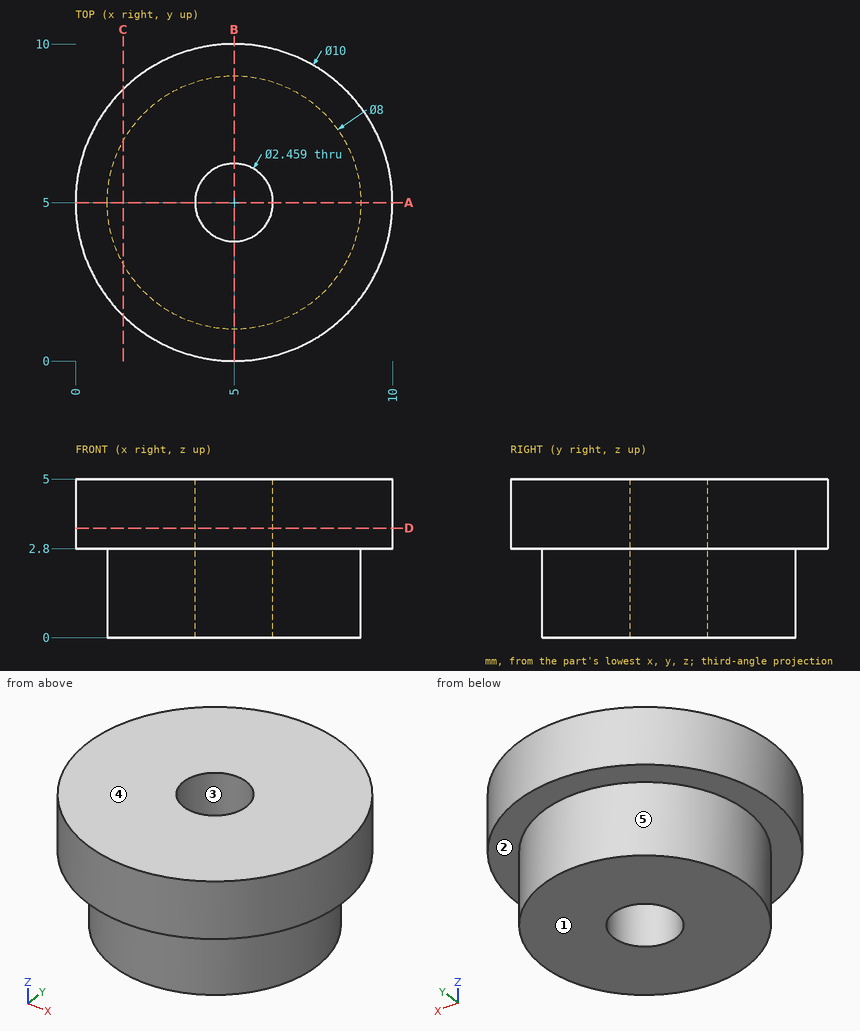
Job drawing, mm, ordinate dimensions from the low corner. One solid piece. A direction names the side the tool comes from. Coordinates: 2 decimals unless noted, no trailing zeros. Loops run counter-clockwise (first coordinate to the right, second up) from the corner with the lowest first, then second, coordinate; pieces in that order, holes last. Notation, with made-up numbers: (73, -26) -> (81, -26) arc R17 ccw to (81, -20) -> close; hole circle Ø1 at (45, 53). An arc over 180 degrees is marked (long way). One line per item, written item: value.
1. Slice it at C-C on x = 1.5. Write the cut outline in (y, z).
Answers:
outline: (1.43, 2.8) -> (3.06, 2.8) -> (3.06, 0) -> (6.94, 0) -> (6.94, 2.8) -> (8.57, 2.8) -> (8.57, 5) -> (1.43, 5) -> close
2. Slice it at A-A on y = 5. Write the cut outline in (x, z), and give its area (3 significant figures).
Answers:
outline: (0, 2.8) -> (1, 2.8) -> (1, 0) -> (3.77, 0) -> (3.77, 5) -> (0, 5) -> close; (6.23, 0) -> (9, 0) -> (9, 2.8) -> (10, 2.8) -> (10, 5) -> (6.23, 5) -> close
area: 32.1 mm^2
3. Pull direction Y, two halves, no side cores. Call the marked faces 3, 4 and 5: pulls with the +Y half, pulls with the -Y half, needs draft (parallel to the pull), parting line crosses it, or undercut.
Answers:
face 3: undercut
face 4: needs draft
face 5: parting line crosses it
4. Which spindle directions (+Z, -Z, +X, -X, +Y, -Y) get a long thin tool onto all of the face, cutting with end or side? Do the marked faces 1 and 2. Say none if no direction does.
Answers:
face 1: -Z, +X, -X, +Y, -Y
face 2: -Z
5. Slice it at D-D on z = 3.45. Write the cut outline in (x, y), and give its area (3 significant figures).
Answers:
outline: circle Ø10 at (5, 5); hole circle Ø2.46 at (5, 5)
area: 73.8 mm^2
6. Flat gauge pins, fed straight in: P1, Ø1.5, axis at y = 7, z = 2.5, coming from the +X side; P2, Ø2, axis at x = 1.5, z = 0.5, coming from the -Y side; P3, Ø1.5, axis at x = 5, y = 5, coming from the +Z side. Where does each tip first touch, or does it go through?
Answers:
P1: stops at x = 9.82
P2: stops at y = 1.88
P3: passes through
7. Drill centre lines: line 1 (Y direction, x = 5, z = 1.75); line 2 (Z direction, x = 9.75, y = 5.25); line 3 (Y direction, x = 5, z = 3.5). Where is each one in solid material? Low to high. Write a range as [from, to].
Answers:
line 1: y = [1, 3.77], [6.23, 9]
line 2: z = [2.8, 5]
line 3: y = [0, 3.77], [6.23, 10]
